```python
from build123d import *

# Parameters (mm, degrees)
F0_W     = 24
F0_H     = 12
F0_W_2   = 1.5
F0_H_2   = 7.7
F1_DEPTH = 0.9
F2_W     = 24
F2_H     = 12
F3_DEPTH = 2.7
F4_R     = 1.6
F5_DEPTH = 1.2
F6_R     = 0.2
F7_R     = 0.8
F8_DEPTH = 5


with BuildPart() as f1:
    # F0 (on Top) → F1 (new body)
    with BuildSketch(Plane.XY):
        Rectangle(F0_W, F0_H)
        Polygon((-10.5, -3.85), (-10.5, 3.85), (-7.5, 3.85), (-6, 3.85), (-3, 3.85), (-1.5, 3.85), (1.5, 3.85), (3, 3.85), (6, 3.85), (7.5, 3.85), (10.5, 3.85), (10.5, -3.85), (7.5, -3.85), (6, -3.85), (3, -3.85), (1.5, -3.85), (-1.5, -3.85), (-3, -3.85), (-6, -3.85), (-7.5, -3.85), align=None, mode=Mode.SUBTRACT)
        with Locations((-6.75, 0)):
            Rectangle(F0_W_2, F0_H_2)
        with Locations((-2.25, 0)):
            Rectangle(F0_W_2, F0_H_2)
        with Locations((2.25, 0)):
            Rectangle(F0_W_2, F0_H_2)
        with Locations((6.75, 0)):
            Rectangle(F0_W_2, F0_H_2)
    extrude(amount=F1_DEPTH)

    # F2 (on face) → F3 (join)
    with BuildSketch(Plane(origin=(0, 0, 0), x_dir=(1, 0, 0), z_dir=(0, 0, -1))):
        Rectangle(F2_W, F2_H)
    extrude(amount=F3_DEPTH)

    # F4 (on face) → F5 (cut)
    with BuildSketch(Plane(origin=(0, 0, -2.7), x_dir=(1, 0, 0), z_dir=(0, 0, -1))):
        Circle(F4_R)
        with Locations((9, 0)):
            Circle(F4_R)
        with Locations((-9, 0)):
            Circle(F4_R)
    extrude(amount=-F5_DEPTH, mode=Mode.SUBTRACT)

    # F6
    f6_edges = [f1.edges().sort_by_distance(p)[0] for p in [
        (-12, -6, -0.9),
        (12, -6, -0.9),
        (12, 6, -0.9),
        (-12, 6, -0.9),
    ]]
    fillet(f6_edges, radius=F6_R)

    # F7 (on face) → F8 (cut)
    with BuildSketch(Plane.XZ.offset(6)):
        with Locations((-6.7, -1.3)):
            Circle(F7_R)
        with Locations((6.7, -1.3)):
            Circle(F7_R)
    extrude(amount=-F8_DEPTH, mode=Mode.SUBTRACT)


solid = f1.part
```
Input: part model. Units: mm. Frame: model coordinates. A direction names the side the tool comes from. Coordinates: 2 decimals unless noted, no trailing zeros. Loops run counter-clockwise (first coordinate to the right, second up) from the corner with the lowest first, then second, coordinate; pieces in that order, holes last. Notation, with made-up numbers: M 82.25,20.25 L 109.25,20.25 A8 ccw 109.25,25.25 Z; hole C 29.25,52 d3. An arc over 180 degrees is marked long. Answer in a Markdown table with one row per item.
1. Section C-C, the plane y = 3. Output: boundary loops of the cut face in (x, z), then the cut area to 3 significant figures.
Response:
| item | result |
|---|---|
| outline | M -12,-2.7 L 12,-2.7 L 12,0.9 L 10.5,0.9 L 10.5,0 L 7.5,0 L 7.5,0.9 L 6,0.9 L 6,0 L 3,0 L 3,0.9 L 1.5,0.9 L 1.5,0 L -1.5,0 L -1.5,0.9 L -3,0.9 L -3,0 L -6,0 L -6,0.9 L -7.5,0.9 L -7.5,0 L -10.5,0 L -10.5,0.9 L -12,0.9 Z |
| area | 72.9 mm2 |
2. Section B-B, the plane x = 9. Output: boundary loops of the cut face in (y, z), then the cut area to 3 significant figures.
Response:
| item | result |
|---|---|
| outline | M -6,-2.7 L -1.6,-2.7 L -1.6,-1.5 L 1.6,-1.5 L 1.6,-2.7 L 6,-2.7 L 6,0.9 L 3.85,0.9 L 3.85,0 L -3.85,0 L -3.85,0.9 L -6,0.9 Z |
| area | 32.4 mm2 |
3. Material intervals for line 1 (X direction, y = 0, z = -2.15); line 2 (X direction, y = 3.5, z = 0.05); line 3 (X direction, y = 1, z = -2.35), sorted ascending.
Response:
| item | result |
|---|---|
| line 1 | x = -12 to -10.6, -7.4 to -1.6, 1.6 to 7.4, 10.6 to 12 |
| line 2 | x = -12 to -10.5, -7.5 to -6, -3 to -1.5, 1.5 to 3, 6 to 7.5, 10.5 to 12 |
| line 3 | x = -12 to -10.25, -7.75 to -1.25, 1.25 to 7.75, 10.25 to 12 |
4. Reachability of faces 1 (the flat face through (-9, 0, -1.5)), 2 (the flat face through (-9, 3.85, 0.4)), 3 (the flat face through (-2.8, 0.1, 0.9)) from +Z, -Z, +X, -X, +Y, -Y: full face, straight path, thin tool, end or side. Return the list, or none.
Response:
| item | result |
|---|---|
| face 1 | -Z |
| face 2 | +Z |
| face 3 | +Z, +X, -X, +Y, -Y |
5. Draft query along X for faces 4 (the flat face through (0, -6, -1)), 5 (the cylindrical face through (7.463, -3.535, -1.06)). Return one class per face: pulls with the +X half, pulls with the -X half, needs draft (parallel to the pull), parting line crosses it, or undercut.
Response:
| item | result |
|---|---|
| face 4 | needs draft |
| face 5 | undercut |
6. Section D-D, the plane x = 4. Output: boundary loops of the cut face in (y, z).
Response:
| item | result |
|---|---|
| outline | M -6,-2.7 L 6,-2.7 L 6,0.9 L 3.85,0.9 L 3.85,0 L -3.85,0 L -3.85,0.9 L -6,0.9 Z |
7. Section A-A, the plane y = -2.25. Output: boundary loops of the cut face in (x, z).
Response:
| item | result |
|---|---|
| outline | M -12,-2.7 L 12,-2.7 L 12,0.9 L 10.5,0.9 L 10.5,0 L 7.5,0 L 7.5,0.9 L 6,0.9 L 6,0 L 3,0 L 3,0.9 L 1.5,0.9 L 1.5,0 L -1.5,0 L -1.5,0.9 L -3,0.9 L -3,0 L -6,0 L -6,0.9 L -7.5,0.9 L -7.5,0 L -10.5,0 L -10.5,0.9 L -12,0.9 Z; hole C -6.7,-1.3 d1.6; hole C 6.7,-1.3 d1.6 |
8. First-contact query: pin 1 (2.5 mm diameter, centred on x = 0, y = 0, fed in from -Z); pin 2 (1.5 mm diameter, centred on x = -8.5, y = 0.5, fed in from +Z); pin 3 (1 mm diameter, centred on x = -6.7, z = -1.3, fed in from -Y). Flat tips, straight axial feed; report the tip coordinate or a pass-through.
Response:
| item | result |
|---|---|
| pin 1 | stops at z = -1.5 |
| pin 2 | stops at z = 0 |
| pin 3 | stops at y = -1 |
